Part model, mm, in its own coordinate system. Round coordinates to 2 decimals unless told otherwise and drop trailing zeros. Write each loop counter-clockwise with the first axis right and the second up, starting at its lowest first coordinate (ties: lowest second). Pieces come first, ordered by that corner, then holes. Notation, with made-up numbers: M 40.5,42 L 62.5,42 A12 ccw 62.5,56 Z; hole C 70.25,3 d8. An arc over 180 degrees is marked long. Use one line per item in the form item = value. Start each with the question number.
Item 1: Probe L1, parallel to Y at x = 5, z = -6.4; L2, parallel to X at y = 7.5, z = -11.15; L3, parallel to Y at x = 7.75, z = 39. List the from-to ranges inside material, lowest first.
Item 2: Flat gauge pins, fed straight in: pin 1 Ø1 at (x, z) = (5.5, -49.5) entering from +Y; pin 2 Ø2.5 at (x, z) = (5.5, 61.5) entering from -Y; pin 3 Ø1.6 at (y, z) = (7.5, -105) entering from +X. Where does each tip first touch, or does it go through?
Item 3: Cut at A-A, the plane z = -6.4. Give the cut face in (x, y), then the cut area to 3 significant figures.
Item 4: Cut at C-C, the plane z = -94.5. Give the cut face in (x, y), then the cut area to 3 significant figures.
Item 5: Cut at B-B, the plane x = 2. Give the cut face in (y, z), then the cut area to 3 significant figures.
from build123d import *

# Parameters (mm, degrees)
SKETCH_1_W               = 120
SKETCH_1_H               = 15
EXTRUDE_1_DEPTH          = 8
FILLET_1_R               = 5
SKETCH_6_R               = 12.5
EXTRUDE_2_DEPTH          = 8
SKETCH_8_R               = 3
CUT_EXTRUDE_5_DEPTH      = 23
SKETCH_9_W               = 8
SKETCH_9_H               = 15
EXTRUDE_3_DEPTH          = 100
SKETCH_10_W              = 50
SKETCH_10_H              = 6
CUT_EXTRUDE_6_DEPTH      = 10
CUT_EXTRUDE_7_DEPTH      = 7
CUT_EXTRUDE_7_DEPTH_BACK = 15
SKETCH_4_R               = 1
FILLET_2_R               = 10
FILLET_4_R               = 5
FILLET_5_R               = 5
SKETCH_11_R              = 1
CUT_EXTRUDE_8_DEPTH      = 10


with BuildPart() as part:
    # 草图1 → 凸台-拉伸1 (new body)
    with BuildSketch(Plane(origin=(0, 0, 0), x_dir=(0, 0, -1), z_dir=(1, 0, 0))):
        with Locations((60, 7.5)):
            Rectangle(SKETCH_1_W, SKETCH_1_H)
    extrude(amount=EXTRUDE_1_DEPTH)

    # 圆角1
    fillet_1_edges = [part.edges().sort_by_distance(p)[0] for p in [
        (4, 15, 0),
        (4, 15, -120),
        (4, 0, -120),
        (4, 0, 0),
    ]]
    fillet(fillet_1_edges, radius=FILLET_1_R)

    # 草图6 → 凸台-拉伸2 (add)
    with BuildSketch(Plane(origin=(8, 0, 0), x_dir=(0, 0, -1), z_dir=(1, 0, 0))):
        with Locations((6.4, 7.5)):
            Circle(SKETCH_6_R)
    extrude(amount=-EXTRUDE_2_DEPTH)

    # 草图8 → 切除-拉伸5 (cut)
    with BuildSketch(Plane.ZY):
        with Locations((-6.4, 7.5)):
            Circle(SKETCH_8_R)
    extrude(amount=-CUT_EXTRUDE_5_DEPTH, mode=Mode.SUBTRACT)

    # 草图9 → 凸台-拉伸3 (add)
    with BuildSketch(Plane.XY):
        with Locations((4, 7.5)):
            Rectangle(SKETCH_9_W, SKETCH_9_H)
    extrude(amount=EXTRUDE_3_DEPTH)

    # 草图10 → 切除-拉伸6 (cut)
    with BuildSketch(Plane.ZY):
        with Locations((28.522995474, 7.5)):
            Rectangle(SKETCH_10_W, SKETCH_10_H)
    extrude(amount=-CUT_EXTRUDE_6_DEPTH, mode=Mode.SUBTRACT)

    # 草图4 → 切除-拉伸7 (cut, two sides: drawn at the far end of the back side and taken through both)
    with BuildSketch(Plane.XY.offset(-CUT_EXTRUDE_7_DEPTH_BACK)):
        with Locations(Location((5, 7.5, 0), (0, 0, 180))):
            Circle(SKETCH_4_R)
    extrude(amount=CUT_EXTRUDE_7_DEPTH + CUT_EXTRUDE_7_DEPTH_BACK, mode=Mode.SUBTRACT)

    # 圆角2
    fillet_2_edges = [part.edges().sort_by_distance(p)[0] for p in [
        (4, 0, -16.4),
        (4, 15, -16.4),
        (4, 15, 3.6),
        (4, 0, 3.6),
    ]]
    fillet(fillet_2_edges, radius=FILLET_2_R)

    # 圆角4
    fillet_4_edges = [part.edges().sort_by_distance(p)[0] for p in [
        (4, 0, 100),
        (4, 15, 100),
    ]]
    fillet(fillet_4_edges, radius=FILLET_4_R)

    # 圆角5
    # the kernel refuses this fillet: 5 mm, written as the material it adds along each edge
    with BuildSketch(Plane(origin=(0, 10.5, 53.522995474), x_dir=(0, 0, -1), z_dir=(1, 0, 0)), Plane(origin=(0, 4.5, 53.522995474), x_dir=(0, 1, 0), z_dir=(1, 0, 0))) as fillet_5_piece_1:
        with BuildLine():
            CenterArc((FILLET_5_R, -FILLET_5_R), FILLET_5_R, 90, 90)
            Line((0, -FILLET_5_R), (0, 0))
            Line((0, 0), (FILLET_5_R, 0))
        make_face()
    extrude(amount=8)

    # 草图11 → 切除-拉伸8 (cut)
    with BuildSketch(Plane.ZY):
        with Locations((-115, 7.5)):
            Circle(SKETCH_11_R)
        with Locations((-105, 7.5)):
            Circle(SKETCH_11_R)
        with Locations((85, 7.5)):
            Circle(SKETCH_11_R)
        with Locations((95, 7.5)):
            Circle(SKETCH_11_R)
    extrude(amount=-CUT_EXTRUDE_8_DEPTH, mode=Mode.SUBTRACT)


solid = part.part
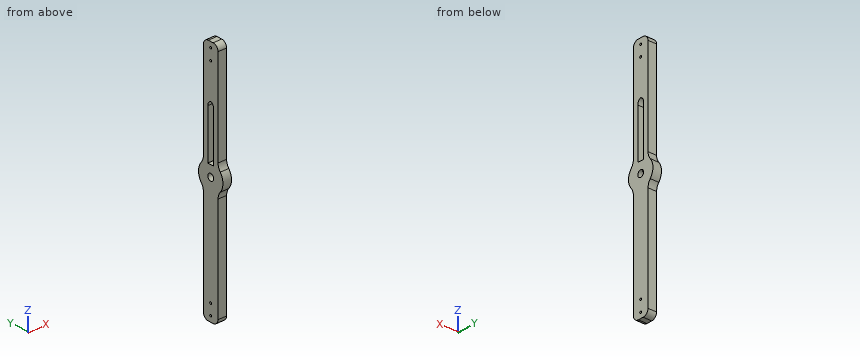
Model answer:
q1.L1 = -5 to 4.5, 10.5 to 20
q1.L2 = 0 to 4, 6 to 8
q1.L3 = 0 to 4.5, 10.5 to 15
q2.pin_1 = 15
q2.pin_2 = 0
q2.pin_3 = through
q3.outline = M 0,-5 L 8,-5 L 8,4.5 L 0,4.5 Z; M 0,10.5 L 8,10.5 L 8,20 L 0,20 Z
q3.area = 152 mm²
q4.outline = M 0,0 L 8,0 L 8,15 L 0,15 Z
q4.area = 120 mm²
q5.outline = M -2.22,-14.26 A10 cw 0,-20.54 L 0,-115 A5 ccw 5,-120 L 10,-120 A5 ccw 15,-115 L 15,-20.54 A10 cw 17.22,-14.26 A12.5 ccw 17.22,1.46 A10 cw 15,7.74 L 15,95 A5 ccw 10,100 L 5,100 A5 ccw 0,95 L 0,7.74 A10 cw -2.22,1.46 A12.5 ccw Z; hole C 7.5,-6.4 d6; hole M 4.5,3.52 L 10.5,3.52 L 10.5,48.52 A5 ccw 7.5,53.11 A5 ccw 4.5,48.52 Z; hole C 7.5,-115 d2; hole C 7.5,-105 d2; hole C 7.5,85 d2; hole C 7.5,95 d2
q5.area = 3,100 mm²
